Geometry check sheet. Reference: the model listing, model coordinates, mm. A direction names the side the tool comes from. Coordinates: 2 decimals unless noted, no trailing zeros. Write each loop counter-clockwise with the first axis right and the second up, starting at its lowest first coordinate (ties: lowest second). Pieces come first, ordered by that corner, then holes. Notation, with made-up numbers: (27.5, -31) -> (44.5, -31) arc R17 cw to (44.5, -17) -> close; hole circle Ø8 at (46, 13.25). An arc over 180 degrees is marked (long way). Answer in a Markdown table with one row per item. Add a question column.
Q1. Section check D-D, the plane z = 32.5. Record the boundary of the cut face in (x, y), and give its area (3 significant figures).
Q2. Section check C-C, the plane z = -9. Record the boundary of the cut face in (x, y), and give its area (3 significant figures).
Q3. Gauge pin test, flat ends, axial feed: P1, Ø6.5, axis at y = -9, z = -21.5, coming from the -X side; P2, Ø0.5, axis at x = -3.5, y = -4, coming from the +Z side; P3, Ø2, axis at x = -28.5, z = -18.5, coming from the -Y side; P4, Ø2, axis at y = -10, z = 36, coming from the +X side (3 decimals). Record the tip position at first contact, or that the pin passes through.
Q4. Thickness scan on line 1 (Y direction, x = 13.5, z = -20); line 2 (Z direction, x = -41, y = -1.25); line 3 (Z direction, x = 57.5, y = -9.75). Record the ranges inside material, lowest first.
Q5. Section check A-A, the plane x = -12. Record the boundary of the cut face in (y, z).
Q6. Section check B-B, the plane y = -3.5. Record the boundary of the cut face in (x, z).
Q7. Tool access check on faces 1 (the face through (4.78, -4, 16)), 2 (the face through (46.759, -6, -18)), 3 (the face through (-1, -12.7, -17)). Record the directions out of +Z, -Z, +X, -X, +Y, -Y that give a thin tool (end or side, any length) a straight path to the whole face; none if there is none.
Q8. Release check for a two-part mould opening along Z. For faces 4 (the face through (-4.087, -4, 16)), 5 (the face through (-1, -13, -52.827)), 6 (the face through (-46.759, -6, -18)) record: pulls with the +Z half, pulls with the -Z half, needs draft (parallel to the pull), parting line crosses it, or undercut.
```python
from build123d import *

# Parameters (mm, degrees)
F0_W     = 135.3589
F0_H     = 25.492367
F1_DEPTH = 25.4
F2_W     = 93.518182
F2_H     = 19.950546
F3_DEPTH = 12.7
F4_W     = 8.866911
F4_H     = 47.382544
F5_DEPTH = 7.62
F6_R     = 16.823006
F7_DEPTH = 7.62


with BuildPart() as f1:
    # F0 (on Front) → F1 (new body)
    with BuildSketch(Plane.XZ):
        with Locations((0, -40.080897)):
            Rectangle(F0_W, F0_H)
    extrude(amount=F1_DEPTH)

    # F2 (on Front) → F3 (join)
    with BuildSketch(Plane.XZ):
        with Locations((0, -17.456727)):
            Rectangle(F2_W, F2_H)
    extrude(amount=F3_DEPTH)

    # F4 (on Front) → F5 (join)
    with BuildSketch(Plane.XZ):
        with Locations((0.346363, 16.209817)):
            Rectangle(F4_W, F4_H)
    extrude(amount=F5_DEPTH)

    # F6 (on Front) → F7 (join)
    with BuildSketch(Plane.XZ):
        with Locations((0, 56.526545)):
            Circle(F6_R)
    extrude(amount=F7_DEPTH)


solid = f1.part
```
Calculated:
| question | item | result |
|---|---|---|
| 1 | outline | (-4.09, -7.62) -> (4.78, -7.62) -> (4.78, 0) -> (-4.09, 0) -> close |
| 1 | area | 67.6 mm² |
| 2 | outline | (-46.76, -12.7) -> (46.76, -12.7) -> (46.76, 0) -> (-46.76, 0) -> close |
| 2 | area | 1,190 mm² |
| 3 | P1 | stops at x = -46.76 |
| 3 | P2 | stops at z = 73.03 |
| 3 | P3 | stops at y = -12.7 |
| 3 | P4 | passes through |
| 4 | line 1 | y = -12.7 to 0 |
| 4 | line 2 | z = -52.83 to -7.48 |
| 4 | line 3 | z = -52.83 to -27.33 |
| 5 | outline | (-25.4, -52.83) -> (0, -52.83) -> (0, -7.48) -> (-12.7, -7.48) -> (-12.7, -27.33) -> (-25.4, -27.33) -> close; (-7.62, 44.74) -> (0, 44.74) -> (0, 68.32) -> (-7.62, 68.32) -> close |
| 6 | outline | (-67.68, -52.83) -> (67.68, -52.83) -> (67.68, -27.33) -> (46.76, -27.33) -> (46.76, -7.48) -> (4.78, -7.48) -> (4.78, 39.9) -> (2.57, 39.9) arc R16.82 ccw (long way) to (-2.57, 39.9) -> (-4.09, 39.9) -> (-4.09, -7.48) -> (-46.76, -7.48) -> (-46.76, -27.33) -> (-67.68, -27.33) -> close |
| 7 | face 1 | +X, +Y, -Y |
| 7 | face 2 | +Z, +X, +Y, -Y |
| 7 | face 3 | +Z, +X, -X, -Y |
| 8 | face 4 | undercut |
| 8 | face 5 | pulls with the -Z half |
| 8 | face 6 | needs draft |
